```python
from build123d import *

# Parameters (mm, degrees)
BOSS_EXTRUDE1_DEPTH             = 238.125
TAP_DRILL_FOR_1_4_20_TAP1_D     = 5.1054
TAP_DRILL_FOR_1_4_20_TAP1_DEPTH = 25.4
TAP_DRILL_FOR_1_4_20_TAP1_TIP   = 1.533816902
TAP_DRILL_FOR_1_4_20_TAP2_D     = 5.1054
TAP_DRILL_FOR_1_4_20_TAP2_DEPTH = 25.4
TAP_DRILL_FOR_1_4_20_TAP2_TIP   = 1.533816902


with BuildPart() as part:
    # Sketch3 → Boss-Extrude1 (new, symmetric)
    with BuildSketch(Plane.XY):
        Polygon((0, 7.332348419), (6.35, 3.666174209), (6.35, -3.666174209), (0, -7.332348419), (-6.35, -3.666174209), (-6.35, 3.666174209), align=None)
    extrude(amount=BOSS_EXTRUDE1_DEPTH, both=True)

    # Tap Drill for 1/4-20 Tap1
    with Locations(Plane.XY.offset(238.125)):
        with Locations((0, 0)):
            Hole(TAP_DRILL_FOR_1_4_20_TAP1_D / 2, depth=TAP_DRILL_FOR_1_4_20_TAP1_DEPTH)
            with Locations((0, 0, -(TAP_DRILL_FOR_1_4_20_TAP1_DEPTH + TAP_DRILL_FOR_1_4_20_TAP1_TIP / 2))):  # 118° drill point
                Cone(0, TAP_DRILL_FOR_1_4_20_TAP1_D / 2, TAP_DRILL_FOR_1_4_20_TAP1_TIP, mode=Mode.SUBTRACT)

    # Tap Drill for 1/4-20 Tap2
    with Locations(Plane(origin=(0, 0, -238.125), x_dir=(-1, 0, 0), z_dir=(0, 0, -1))):
        with Locations((0, 0)):
            Hole(TAP_DRILL_FOR_1_4_20_TAP2_D / 2, depth=TAP_DRILL_FOR_1_4_20_TAP2_DEPTH)
            with Locations((0, 0, -(TAP_DRILL_FOR_1_4_20_TAP2_DEPTH + TAP_DRILL_FOR_1_4_20_TAP2_TIP / 2))):  # 118° drill point
                Cone(0, TAP_DRILL_FOR_1_4_20_TAP2_D / 2, TAP_DRILL_FOR_1_4_20_TAP2_TIP, mode=Mode.SUBTRACT)


solid = part.part
```
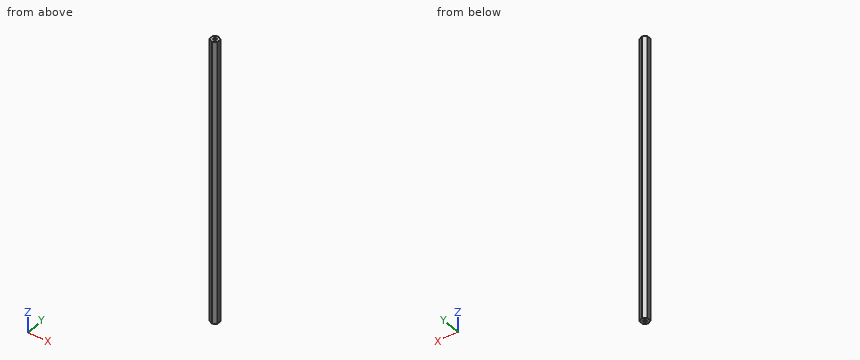
Could you check a few things on this model? Use its own coordinates, in mm. Round coordinates to 2 decimals unless told otherwise and drop trailing zeros. Loops run counter-clockwise (first coordinate to the right, second up) from the corner with the lowest first, then second, coordinate; pieces in that order, holes last. Notation, with made-up numbers: (48.25, 12.5) -> (107.25, 12.5) arc R25 cw to (107.25, 34.5) -> close; hole circle Ø1 at (-24.5, -1). An arc over 180 degrees is marked (long way). One line per question, with ' | ' between items.
(1) If we section it at A-A on z = 94.5: List the corners of the cut face in (x, y) for me.
Model answer:
outline: (-6.35, -3.67) -> (0, -7.33) -> (6.35, -3.67) -> (6.35, 3.67) -> (0, 7.33) -> (-6.35, 3.67) -> close
(2) For pin 1 Ø5 at (y, z) = (4.5, 96) entering from -X; pin 2 Ø1 at (y, z) = (-5, -54.5) entering from +X; pin 3 Ø2 at (x, z) = (4, 112) entering from -Y; pin 4 Ø4.5 at (x, y) = (0, 0) entering from +Z, each with a flat end and sliding along its axis, tell me the tip position at first contact or that it passes through.
Model answer:
pin 1: stops at x = -6.35 | pin 2: stops at x = 4.91 | pin 3: stops at y = -5.6 | pin 4: stops at z = 212.54
(3) If I drill on probe 1 along Y at (x, z) = (0, -227.75); probe 2 along X at (y, z) = (0, -219.75); probe 3 along Y at (x, z) = (1.75, -177.5), over which ranges is the centre line in solid material (lowest first)?
Model answer:
probe 1: y = -7.33 to -2.55, 2.55 to 7.33 | probe 2: x = -6.35 to -2.55, 2.55 to 6.35 | probe 3: y = -6.32 to 6.32
